from build123d import *

# Parameters (mm, degrees)
CROQUIS1_R              = 2
SALIENTE_EXTRUIR5_DEPTH = 5


with BuildPart() as part:
    # Croquis1 → Saliente-Extruir5 (new body)
    with BuildSketch(Plane.XY):
        with BuildLine():
            Line((-7.5, -40), (-7.5, 0))
            ThreePointArc((-7.5, 0), (0, 7.5), (7.5, 0))
            Line((7.5, 0), (7.5, -40))
            Line((7.5, -40), (2.499716416, -127.5))
            Line((2.499716416, -127.5), (2.499716416, -132.5))
            Line((2.499716416, -132.5), (-2.499716416, -132.5))
            Line((-2.499716416, -132.5), (-2.499716416, -127.5))
            Line((-2.499716416, -127.5), (-7.5, -40))
        make_face()
        with Locations((0, -38)):
            Circle(CROQUIS1_R, mode=Mode.SUBTRACT)
        Circle(CROQUIS1_R, mode=Mode.SUBTRACT)
    extrude(amount=SALIENTE_EXTRUIR5_DEPTH)


solid = part.part
Part model, mm, in its own coordinate system. A direction names the side the tool comes from. Round coordinates to 2 decimals unless told otherwise and drop trailing zeros. Write each loop counter-clockwise with the first axis right and the second up, starting at its lowest first coordinate (ties: lowest second). Pieces come first, ordered by that corner, then holes. Notation, with made-up numbers: M 84.25,-3 L 132.25,-3 A16 cw 132.25,26 Z; hole C 24.5,46 d8. An arc over 180 degrees is marked long. Return JSON: item names as keys, results as strings. Group by question number.
(1) Drill centre lines: probe 1 along Y at (x, z) = (0, 1); probe 2 along Y at (x, z) = (0.75, 3.4); probe 3 along X at (y, z) = (-118, 3.45). Where is each one in solid material? Low to high.
(2) Saw through at B-B on y = -38. Write the cut outline in (x, z).
(3) Saw through at A-A on x = 0. Write the cut outline in (y, z).
(4) Two-plate mould, pull along X, no slides. Class faces 1 (the face through (0, -2, 2)), 2 (the face through (2.5, -130, 2)), 3 (the face through (0, -46, 0)), 4 (the face through (0, -40, 2)): +X half, -X half, draft (parallel to the pull), parting line (faces both ways), or undercut.
(5) Saw through at C-C on z = 0.95. Write the cut outline in (x, y), then the cut area to 3 significant figures.
(6) Which spindle directions (+Z, -Z, +X, -X, +Y, -Y) get a long thin tool onto all of the face, cutting with end or side? Do faces 5 (the face through (0, -46, 5)), 6 (the face through (-2.5, -130, 2)). Say none if no direction does.
(7) Saw through at D-D on y = -77. Write the cut outline in (x, z).
(8) Pin check, flat tips, straight feed: pin 1 Ø3 at (y, z) = (-60.5, 1) entering from +X; pin 2 Ø2.5 at (y, z) = (-129, 2.5) entering from +X. Stop position of each tip, or through.
Returned:
{
 "1": {"probe 1": "-132.5 to -40, -36 to -2, 2 to 7.5", "probe 2": "-132.5 to -39.85, -36.15 to -1.85, 1.85 to 7.46", "probe 3": "-3.04 to 3.04"},
 "2": {"outline": "M -7.5,0 L -2,0 L -2,5 L -7.5,5 Z; M 2,0 L 7.5,0 L 7.5,5 L 2,5 Z"},
 "3": {"outline": "M -132.5,0 L -40,0 L -40,5 L -132.5,5 Z; M -36,0 L -2,0 L -2,5 L -36,5 Z; M 2,0 L 7.5,0 L 7.5,5 L 2,5 Z"},
 "4": {"face 1": "undercut", "face 2": "+X half", "face 3": "draft", "face 4": "undercut"},
 "5": {"outline": "M -7.5,-40 L -2.5,-127.5 L -2.5,-132.5 L 2.5,-132.5 L 2.5,-127.5 L 7.5,-40 L 7.5,0 A7.5 ccw -7.5,0 Z; hole C 0,-38 d4; hole C 0,0 d4", "area": "1,560 mm²"},
 "6": {"face 5": "+Z, +X, -X, +Y, -Y", "face 6": "+Z, -Z, -X, -Y"},
 "7": {"outline": "M -5.39,0 L 5.39,0 L 5.39,5 L -5.39,5 Z"},
 "8": {"pin 1": "x = 6.41", "pin 2": "x = 2.5"}
}
